```python
from build123d import *

# Parameters (mm, degrees)
MODEL_R                  = 1.500000022
MODEL_W                  = 5.000000119
MODEL_H                  = 5.000000119
MODEL_H_2                = 8.000000119
MODEL_H_3                = 11.000000119
MODEL_H_4                = 10
RESSALTO_EXTRUS_O1_DEPTH = 5


with BuildPart() as part:
    # Model → Ressalto-extrusão1 (new body)
    with BuildSketch(Plane.XY):
        with BuildLine():
            Line((-180.698726154, 44.000000686), (-209.539314988, 44.000000686))
            ThreePointArc((-209.539314988, 44.000000686), (-211.26607554, 44.278095095), (-212.818217016, 45.084255959))
            ThreePointArc((-212.818217016, 45.084255959), (-236.218705268, 59.378884867), (-261.807031602, 69.235700855))
            ThreePointArc((-261.807031602, 69.235700855), (-264.518550223, 69.808004431), (-267.283148189, 70.000001046))
            Line((-267.283148189, 70.000001046), (-355.903623858, 70.000001046))
            ThreePointArc((-355.903623858, 70.000001046), (-372.979904567, 77.073228111), (-380.053131631, 94.149508819))
            Line((-380.053131631, 94.149508819), (-380.053131631, 94.691449457))
            ThreePointArc((-380.053131631, 94.691449457), (-372.93332153, 111.880191563), (-355.744579423, 119.000001664))
            Line((-355.744579423, 119.000001664), (-268.169073012, 119.000001664))
            ThreePointArc((-268.169073012, 119.000001664), (-264.984221388, 119.255211968), (-261.880650458, 120.014329651))
            ThreePointArc((-261.880650458, 120.014329651), (-236.634658237, 130.102883651), (-212.786381277, 143.156570145))
            ThreePointArc((-212.786381277, 143.156570145), (-211.382514446, 143.784939438), (-209.859544299, 144.000002169))
            Line((-209.859544299, 144.000002169), (-180.698726151, 144.000002169))
            ThreePointArc((-180.698726151, 144.000002169), (-177.244327452, 143.215757822), (-174.467201918, 141.016784577))
            ThreePointArc((-174.467201918, 141.016784577), (-157.893223845, 94.000001427), (-174.467201921, 46.983218277))
            ThreePointArc((-174.467201921, 46.983218277), (-177.244327455, 44.784245034), (-180.698726154, 44.000000686))
        make_face()
        with Locations((-281.500004195, 112.000001669)):
            Circle(MODEL_R, mode=Mode.SUBTRACT)
        with Locations((-184.500002749, 124.500001855)):
            Circle(MODEL_R, mode=Mode.SUBTRACT)
        with Locations((-251.500003748, 112.000001669)):
            Circle(MODEL_R, mode=Mode.SUBTRACT)
        with Locations((-236.500003524, 112.000001669)):
            Circle(MODEL_R, mode=Mode.SUBTRACT)
        with Locations((-266.500003971, 112.000001669)):
            Circle(MODEL_R, mode=Mode.SUBTRACT)
        with Locations((-281.499999941, 105.500001595)):
            Rectangle(MODEL_W, MODEL_H, mode=Mode.SUBTRACT)
        with Locations((-281.499999941, 83.000001236)):
            Rectangle(MODEL_W, MODEL_H_2, mode=Mode.SUBTRACT)
        with Locations((-236.50000006, 105.500001595)):
            Rectangle(MODEL_W, MODEL_H, mode=Mode.SUBTRACT)
        with Locations((-236.50000006, 83.000001236)):
            Rectangle(MODEL_W, MODEL_H_2, mode=Mode.SUBTRACT)
        with Locations((-251.499999941, 83.000001236)):
            Rectangle(MODEL_W, MODEL_H_2, mode=Mode.SUBTRACT)
        with Locations((-251.499999941, 105.500001595)):
            Rectangle(MODEL_W, MODEL_H, mode=Mode.SUBTRACT)
        with Locations((-184.499999941, 69.500001367)):
            Rectangle(MODEL_W, MODEL_H_3, mode=Mode.SUBTRACT)
        with Locations((-184.499999941, 136.000001903)):
            Rectangle(MODEL_W, MODEL_H_4, mode=Mode.SUBTRACT)
        with Locations((-184.499999941, 114.000001664)):
            Rectangle(MODEL_W, MODEL_H_4, mode=Mode.SUBTRACT)
        with Locations((-266.499999941, 83.000001236)):
            Rectangle(MODEL_W, MODEL_H_2, mode=Mode.SUBTRACT)
        with Locations((-266.499999941, 105.500001595)):
            Rectangle(MODEL_W, MODEL_H, mode=Mode.SUBTRACT)
        with BuildLine():
            Line((-362.000002593, 91.000001416), (-169.000002593, 91.000001416))
            ThreePointArc((-169.000002593, 91.000001416), (-165.000002841, 95.000001167), (-169.000002593, 99.000000919))
            Line((-169.000002593, 99.000000919), (-362.000002593, 99.000000919))
            ThreePointArc((-362.000002593, 99.000000919), (-366.000002344, 95.000001167), (-362.000002593, 91.000001416))
        make_face(mode=Mode.SUBTRACT)
    extrude(amount=RESSALTO_EXTRUS_O1_DEPTH)


solid = part.part
```
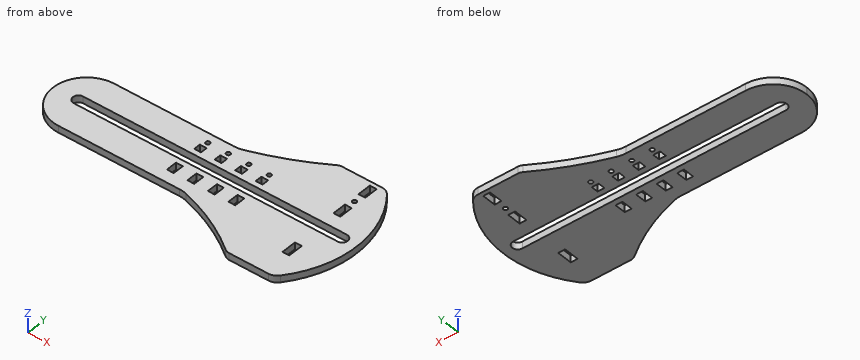
Check sheet for the modelled part. Datum: model origin and axes. Units: mm. Give positions to 0.01 mm unless a question says otherwise; leave off trailing zeros. Order: outer loops, then holes, each group sorted by start corner. A loop starts at its lowest first (then second) coordinate and runs counter-clockwise, first axis right, second up. Notation, with made-up numbers: (77.5, 3.25) -> (114.5, 3.25) arc R20 ccw to (114.5, 41.25) -> close; hole circle Ø3 at (77.5, -2). An arc over 180 degrees is marked (long way). Return JSON: item names as keys, results as strings.
1. Go/stop test with flat-tipped pins: P1, Ø2.5, axis at y = 81.5, z = 1.5, coming from the -X side; P2, Ø2.5, axis at x = -281.5, y = 112, coming from the -Z side; P3, Ø2, axis at x = -252, z = 3, coming from the +Y side; P4, Ø1.5, axis at x = -280.5, z = 3.5, coming from the -Y side. Record where each tip stops, or that it passes through.
From the geometry:
{"P1": "x = -377.19", "P2": "through", "P3": "y = 123.93", "P4": "y = 70"}
2. Material ranges on probe 1 along Y at (x, z) = (-186.5, 3.65); probe 2 along Y at (x, z) = (-276, 4.2); probe 3 along X at (y, z) = (81, 3.95), recorded low to high. Write a range as [from, to].
From the geometry:
{"probe 1": "[44, 64], [75, 91], [99, 109], [119, 131], [141, 144]", "probe 2": "[70, 91], [99, 119]", "probe 3": "[-376.16, -284], [-279, -269], [-264, -254], [-249, -239], [-234, -159.03]"}
3. Cross-section at C-C, the plane z = 1.6. Count the separate pieces of the cut face and the enclosed holes in it, plus the area to 3 significant figures.
From the geometry:
{"separate pieces": "1", "enclosed holes": "17", "area": "11,900 mm^2"}
4. Cross-section at A-A, the plane x = -201. Record the cut outline in (y, z).
From the geometry:
{"outline": "(44, 0) -> (91, 0) -> (91, 5) -> (44, 5) -> close; (99, 0) -> (144, 0) -> (144, 5) -> (99, 5) -> close"}
5. Cross-section at B-B, the plane y = 133. Record the cut outline in (x, z).
From the geometry:
{"outline": "(-230.71, 0) -> (-187, 0) -> (-187, 5) -> (-230.71, 5) -> close; (-182, 0) -> (-168.83, 0) -> (-168.83, 5) -> (-182, 5) -> close"}
